The model under review builds one solid part; all positions refer to its coordinate system, in mm. A direction names the side the tool comes from. Coordinates: 2 decimals unless noted, no trailing zeros. Order: outer loops, then holes, each group sorted by start corner. A loop starts at its lowest first (then second) coordinate and runs counter-clockwise, first axis right, second up.
```python
from build123d import *

# Parameters (mm, degrees)
SKETCH1_W           = 15
SKETCH1_H           = 55
SKETCH1_R           = 1.5
SKETCH1_W_2         = 30
SKETCH1_H_2         = 20
SKETCH1_R_2         = 2.55
BOSS_EXTRUDE1_DEPTH = 10


with BuildPart() as part:
    # Sketch1 → Boss-Extrude1 (new body)
    # profile 1 of 2: a face of its own
    with BuildSketch(Plane(origin=(0, 0, 0), x_dir=(1, 0, 0), z_dir=(0, 1, 0))):
        Rectangle(SKETCH1_W, SKETCH1_H)
        with Locations(Location((0, -22.5, 0), (0, 0, 270))):
            Circle(SKETCH1_R, mode=Mode.SUBTRACT)
        with Locations(Location((0, 17.5, 0), (0, 0, 270))):
            Circle(SKETCH1_R, mode=Mode.SUBTRACT)
    # profile 2 of 2: a face of its own
    with BuildSketch(Plane(origin=(0, 0, 0), x_dir=(1, 0, 0), z_dir=(0, 1, 0))):
        with Locations((-22.5, 17.5)):
            Rectangle(SKETCH1_W_2, SKETCH1_H_2)
        with Locations(Location((-29.5, 17.5, 0), (0, 0, 270))):
            Circle(SKETCH1_R_2, mode=Mode.SUBTRACT)
    extrude(amount=BOSS_EXTRUDE1_DEPTH)


solid = part.part
```
(1) We need section A-A, the plane z = -17.5. Write out the cut boundary in (x, y), and give its area (3 significant figures).
A:
outline: (-37.5, 0) - (-32.05, 0) - (-32.05, 10) - (-37.5, 10) - close; (-26.95, 0) - (-1.5, 0) - (-1.5, 10) - (-26.95, 10) - close; (1.5, 0) - (7.5, 0) - (7.5, 10) - (1.5, 10) - close
area: 369 mm2
(2) For pin 1 Ø4 at (y, z) = (4.5, 9.5) entering from -X; pin 2 Ø2 at (x, z) = (-10, 16.5) entering from -Y; pin 3 Ø6 at (x, y) = (-13.5, 8.5) entering from +Z, all flat-tipped, find the tip position at first contact; note any pin that passes through.
A:
pin 1: stops at x = -7.5
pin 2: passes through
pin 3: stops at z = -7.5
(3) We need section D-D, the plane z = 22.5. Write out the cut boundary in (x, y), and give its area (3 significant figures).
A:
outline: (-7.5, 0) - (-1.5, 0) - (-1.5, 10) - (-7.5, 10) - close; (1.5, 0) - (7.5, 0) - (7.5, 10) - (1.5, 10) - close
area: 120 mm2
(4) Wall thickness on probe 1 along X at (y, z) = (5, -17.5); probe 2 along X at (y, z) = (7.5, 22.5); probe 3 along Z at (x, y) = (0.5, 6.25): over which ranges is each line inside the solid? List them lowest first.
A:
probe 1: x = -37.5 to -32.05, -26.95 to -1.5, 1.5 to 7.5
probe 2: x = -7.5 to -1.5, 1.5 to 7.5
probe 3: z = -27.5 to -18.91, -16.09 to 21.09, 23.91 to 27.5
(5) We need section C-C, the plane x = -29.5. Write out the cut boundary in (y, z).
A:
outline: (0, -27.5) - (10, -27.5) - (10, -20.05) - (0, -20.05) - close; (0, -14.95) - (10, -14.95) - (10, -7.5) - (0, -7.5) - close
(6) Draft analysis for pull direction Z (two halves, no side actions). For faces 1 (the face through (0, 5, -19)), 2 (the face through (-15, 5, -27.5)), 3 (the face through (-5, 10, -6)), state which applies: released by +Z, released by -Z, zero draft, split by the parting line, or undercut.
A:
face 1: undercut
face 2: released by -Z
face 3: zero draft
(7) Machinability: for faces 4 (the face through (-7.5, 5, 10)), 5 (the face through (-37.5, 5, -17)), which of the approach directions +Z, -Z, +X, -X, +Y, -Y give a long, thin tool a straight path to every point of the face, cutting with its end or side? Answer none if there is none.
A:
face 4: +Z, -X, +Y, -Y
face 5: +Z, -Z, -X, +Y, -Y
(8) We need section B-B, the plane y = 7.5. Write out the cut boundary in (x, z).
A:
outline: (-37.5, -27.5) - (7.5, -27.5) - (7.5, 27.5) - (-7.5, 27.5) - (-7.5, -7.5) - (-37.5, -7.5) - close; hole circle Ø5.1 at (-29.5, -17.5); hole circle Ø3 at (0, -17.5); hole circle Ø3 at (0, 22.5)
